Read the model definition and answer for the solid it produces. Units are mm, in the model's axes. Give positions to 0.01 mm unless a question says otherwise; leave off trailing zeros. Loops run counter-clockwise (first coordinate to the right, second up) from the corner with the lowest first, then second, coordinate; pieces in that order, holes last. Notation, with made-up numbers: (7, 12.5) - (26, 12.5) arc R16 ccw to (26, 35.5) - close; hole circle Ø11 at (-27, 48.25). An arc over 180 degrees is marked (long way). Use a Markdown table: item, result. Add a question column.
Item 1: A cutting plane is placed at D-D (z = -22.5). Determine the outline of the cut face in (x, y), plus the area to 3 significant figures.
Item 2: A cutting plane is placed at B-B (x = -12). Determine the outline of the cut face in (y, z), plus the area to 3 significant figures.
Item 3: A cutting plane is placed at A-A (z = 0). Determine the outline of the cut face in (x, y).
Item 4: Consider probe 1 along X at (y, z) = (1.5, 18); probe 2 along Z at (x, y) = (16, -5); probe 3 along Z at (x, y) = (16, -4.5). Determine where each line is inside the solid, lowest interval first. Write a range as [from, to].
Item 5: A cutting plane is placed at C-C (y = 5.5). Determine the outline of the cut face in (x, z), plus the area to 3 significant figures.
Item 6: For a pull along X with two mould halves and no side action, classify faces 1 (the face through (16.363, 1.517, -1.121)), 2 (the face through (-0.382, -3.774, -25.982)), 3 (the face through (16.363, -1.517, -1.121)), 4 (the face through (-26.49, 0.05, 26.96)) as +X half, -X half, draft (parallel to the pull), parting line (faces both ways), or undercut.
Item 7: Each of these flat-tipped pins is pushed along its axis until it touches: P1, Ø2, axis at x = -11, y = -5, coming from the +Z side; P2, Ø2, axis at y = 3, z = 20, coming from the -X side; P3, Ø2, axis at x = 20.5, y = -4, coming from the +Z side. Where does it stop, or does it pass through?
from build123d import *

# Parameters (mm, degrees)
F0_W        = 55.88
F0_H        = 56.9722
F0_R        = 2.6797
F1_DEPTH    = 6.35
F2_R        = 5.08
F3_R        = 5.08
F4_T1_DEPTH = 71.8482991577
F5_T1_DEPTH = 71.8482991577


# Not quite as in the source:
# - a fillet or chamfer that OpenCascade refuses, or shapes differently, is made with other operations: its cross-section is extruded or revolved along the edge and cut away or added


with BuildPart() as f1:
    # F0 (on Front) → F1 (new body, symmetric)
    with BuildSketch(Plane.XZ):
        Rectangle(F0_W, F0_H)
        with Locations((13.660245575, 0)):
            Circle(F0_R, mode=Mode.SUBTRACT)
    extrude(amount=F1_DEPTH, both=True)

    # F2
    f2_edges = [f1.edges().sort_by_distance(p)[0] for p in [
        (-27.94, 6.35, 0),
        (-27.94, 0, -28.4861),
        (-27.94, -6.35, 0),
        (-27.94, 0, 28.4861),
    ]]
    fillet(f2_edges, radius=F2_R)

    # F3
    f3_edges = [f1.edges().sort_by_distance(p)[0] for p in [
        (27.94, 0, -28.4861),
        (27.94, 6.35, 0),
        (27.94, 0, 28.4861),
        (27.94, -6.35, 0),
    ]]
    fillet(f3_edges, radius=F3_R)

    # F4: chamfer of 5.08 on 5 edges, made by hand

    # F4_s2 → F4_t1 (cut)
    with BuildSketch(Plane.YZ.offset(-35.9241495789)):
        Polygon((-1.27, -28.4861), (-6.35, -23.4061), (-6.35, -28.4861), align=None)
        Polygon((-6.35, 23.4061), (-1.27, 28.4861), (-6.35, 28.4861), align=None)
    extrude(amount=F4_T1_DEPTH, mode=Mode.SUBTRACT)

    # F4_s3 → F4_t4 (revolve, cut)
    with BuildSketch(Plane.XY):
        Polygon((21.419945575, -6.35), (16.339945575, -1.27), (16.339945575, -6.35), align=None)
    revolve(axis=Axis((13.660245575, -6.35, 0), (0, -1, 0)), mode=Mode.SUBTRACT)

    # F5: chamfer of 5.08 on 5 edges, made by hand

    # F5_s2 → F5_t1 (cut)
    with BuildSketch(Plane.YZ.offset(-35.9241495789)):
        Polygon((1.27, -28.4861), (6.35, -23.4061), (6.35, -28.4861), align=None)
        Polygon((6.35, 23.4061), (1.27, 28.4861), (6.35, 28.4861), align=None)
    extrude(amount=F5_T1_DEPTH, mode=Mode.SUBTRACT)

    # F5_s3 → F5_t4 (revolve, cut)
    with BuildSketch(Plane.XY):
        Polygon((21.419945575, 6.35), (16.339945575, 1.27), (16.339945575, 6.35), align=None)
    revolve(axis=Axis((13.660245575, 6.35, 0), (0, -1, 0)), mode=Mode.SUBTRACT)


solid = f1.part
Geometry says:
| question | item | result |
|---|---|---|
| 1 | outline | (-27.94, -1.27) arc R5.08 ccw to (-22.86, -6.35) - (22.86, -6.35) arc R5.08 ccw to (27.94, -1.27) - (27.94, 1.27) arc R5.08 ccw to (22.86, 6.35) - (-22.86, 6.35) arc R5.08 ccw to (-27.94, 1.27) - close |
| 1 | area | 688 mm² |
| 2 | outline | (-6.35, -23.41) - (-1.27, -28.49) - (1.27, -28.49) - (6.35, -23.41) - (6.35, 23.41) - (1.27, 28.49) - (-1.27, 28.49) - (-6.35, 23.41) - close |
| 2 | area | 672 mm² |
| 3 | outline | (-27.94, -1.27) arc R5.08 ccw to (-22.86, -6.35) - (5.9, -6.35) - (10.98, -1.27) - (10.98, 1.27) - (5.9, 6.35) - (-22.86, 6.35) arc R5.08 ccw to (-27.94, 1.27) - close; (16.34, -1.27) - (21.42, -6.35) - (22.86, -6.35) arc R5.08 ccw to (27.94, -1.27) - (27.94, 1.27) arc R5.08 ccw to (22.86, 6.35) - (21.42, 6.35) - (16.34, 1.27) - close |
| 4 | probe 1 | [-27.93, 27.93] |
| 4 | probe 2 | [-24.76, -5.97], [5.97, 24.76] |
| 4 | probe 3 | [-25.26, -5.43], [5.43, 25.26] |
| 5 | outline | (-25.67, -24.26) - (25.67, -24.26) - (25.67, 24.26) - (-25.67, 24.26) - close; hole circle Ø13.82 at (13.66, 0) |
| 5 | area | 2,340 mm² |
| 6 | face 1 | undercut |
| 6 | face 2 | draft |
| 6 | face 3 | undercut |
| 6 | face 4 | -X half |
| 7 | P1 | z = 25.76 |
| 7 | P2 | x = -27.89 |
| 7 | P3 | z = 26.76 |
